```python
from build123d import *

# Parameters (mm, degrees)
F0_R     = 3.571875
F0_R_2   = 3.175
F0_R_3   = 2.778125
F0_R_4   = 2.38125
F0_R_5   = 1.984375
F0_R_6   = 1.5875
F0_R_7   = 3.96875
F0_R_8   = 4.365625
F0_R_9   = 4.7625
F0_R_10  = 5.159375
F0_R_11  = 5.55625
F0_R_12  = 6.35
F1_DEPTH = 3.175


# Not quite as in the source:
# - a length typed as a fraction of an inch, garbled in the dataset ("3 / 203.2 mm" for 3/8 in), is restored


with BuildPart() as f1:
    # F0 (on Front) → F1 (new body)
    with BuildSketch(Plane.XZ):
        with BuildLine():
            Line((0, 50.8), (0, 0))
            Line((0, 0), (120.65, 0))
            ThreePointArc((120.65, 0), (125.1401280605, 1.8598719395), (127, 6.35))
            Line((127, 6.35), (127, 44.45))
            ThreePointArc((127, 44.45), (125.1401280605, 48.9401280605), (120.65, 50.8))
            Line((120.65, 50.8), (0, 50.8))
        make_face()
        with Locations((13.97, 10.5871595442)):
            Circle(F0_R, mode=Mode.SUBTRACT)
        with Locations((32.766, 10.5871595442)):
            Circle(F0_R_2, mode=Mode.SUBTRACT)
        with Locations((51.562, 10.5871595442)):
            Circle(F0_R_3, mode=Mode.SUBTRACT)
        with Locations((70.358, 10.5871595442)):
            Circle(F0_R_4, mode=Mode.SUBTRACT)
        with Locations((89.154, 10.5871595442)):
            Circle(F0_R_5, mode=Mode.SUBTRACT)
        with Locations((107.95, 10.5871595442)):
            Circle(F0_R_6, mode=Mode.SUBTRACT)
        with Locations((12.7109313135, 39.5430161922)):
            Circle(F0_R_7, mode=Mode.SUBTRACT)
        with Locations((31.7587450508, 39.2544129538)):
            Circle(F0_R_8, mode=Mode.SUBTRACT)
        with Locations((50.8065587881, 38.9658097153)):
            Circle(F0_R_9, mode=Mode.SUBTRACT)
        with Locations((69.8543725254, 38.6772064769)):
            Circle(F0_R_10, mode=Mode.SUBTRACT)
        with Locations((88.9021862627, 38.3886032384)):
            Circle(F0_R_11, mode=Mode.SUBTRACT)
        with Locations((107.95, 38.1)):
            Circle(F0_R_12, mode=Mode.SUBTRACT)
        with BuildLine():
            ThreePointArc((0, 50.8), (-25.4, 25.4), (0, 0))
            Line((0, 0), (0, 50.8))
        make_face()
    extrude(amount=F1_DEPTH)


solid = f1.part
```
Here's how the part is built. I have some questions about the finished solid (model axes, mm). Round coordinates to 2 decimals unless told otherwise and drop trailing zeros. Loops run counter-clockwise (first coordinate to the right, second up) from the corner with the lowest first, then second, coordinate; pieces in that order, holes last. Notation, with made-up numbers: (18.5, 28) -> (25.5, 28) arc R12 cw to (25.5, 45) -> close; hole circle Ø1 at (10, -20.5). An arc over 180 degrees is marked (long way). Answer as CSV lines item,"result".
1. For pin 1 (5 mm diameter, centred on x = 32.77, z = 10.59, fed in from +Y); pin 2 (1.5 mm diameter, centred on y = -1, z = 8.5, fed in from -X), each with a flat end and sliding along its axis, tell me the tip position at first contact or that it passes through.
Final values:
pin 1,"passes through"
pin 2,"stops at x = -19.6"
2. If I drill on L1, parallel to Z at x = 107.95, y = -1.85; L2, parallel to Z at x = 15, y = -2; L3, parallel to Z at x = 110.5, y = -0.4, over which ranges is the centre line in solid material (lowest first)?
Final values:
L1,"z = 0 to 9, 12.17 to 31.75, 44.45 to 50.8"
L2,"z = 0 to 7.17, 14.01 to 36.3, 42.79 to 50.8"
L3,"z = 0 to 32.28, 43.92 to 50.8"
3. If we section it at A-A on x = 107.95: Please give me the cut outline in (y, z) (3 decimals).
Final values:
outline,"(-3.175, 0) -> (0, 0) -> (0, 9) -> (-3.175, 9) -> close; (-3.175, 12.175) -> (0, 12.175) -> (0, 31.75) -> (-3.175, 31.75) -> close; (-3.175, 44.45) -> (0, 44.45) -> (0, 50.8) -> (-3.175, 50.8) -> close"
4. If we section it at B-B on y = -1: Count the separate pieces of the cut face and the enclosed holes in it, plus the area to 3 significant figures.
Final values:
separate pieces,"1"
enclosed holes,"12"
area,"6,830 mm^2"
5. Thinking about a two-plate mould opening in X: for faces 1 (the face through (59, -2, 0)), 2 (the face through (-25.394, -1.565, 25.959)), 3 (the face through (102.91, -1.57, 34.24)), which applies, released by +X, released by -X, zero draft, split by the parting line, or undercut?
Final values:
face 1,"zero draft"
face 2,"released by -X"
face 3,"undercut"
